```python
from build123d import *

# Parameters (mm, degrees)
SKETCH_W        = 10
SKETCH_H        = 6
PAD_DEPTH       = 3
SKETCH001_R     = 1.1
POCKET_DEPTH    = 6.001
SKETCH002_R     = 0.5
POCKET001_DEPTH = 1
CHAMFER_SIZE    = 1.2
SKETCH004_R     = 0.6
POCKET002_DEPTH = 6.001
FILLET_R        = 0.5
CHAMFER001_SIZE = 0.2


with BuildPart() as part:
    # Sketch → Pad (new body, symmetric)
    with BuildSketch(Plane.XY):
        with Locations((-5, 0)):
            Rectangle(SKETCH_W, SKETCH_H)
    extrude(amount=PAD_DEPTH, both=True)

    # Sketch001 (on Face6 of Pad) → Pocket (cut, through all)
    with BuildSketch(Plane.XY.offset(3)):
        with Locations((-5, 0)):
            Circle(SKETCH001_R)
    extrude(amount=-POCKET_DEPTH, mode=Mode.SUBTRACT)

    # Sketch002 (on Face1 of Pocket) → Pocket001 (cut)
    with BuildSketch(Plane.XZ.offset(3)):
        with Locations((-8.5, 0)):
            Circle(SKETCH002_R)
    extrude(amount=-POCKET001_DEPTH, mode=Mode.SUBTRACT)

    # Chamfer
    chamfer_edges = [part.edges().sort_by_distance(p)[0] for p in [
        (-6.1, 0, 3),
    ]]
    chamfer(chamfer_edges, length=CHAMFER_SIZE)

    # Sketch004 (on Face3 of Chamfer) → Pocket002 (cut, through all)
    with BuildSketch(Plane.XZ.offset(3)):
        with Locations((-8.5, 1.75)):
            Circle(SKETCH004_R)
        with Locations((-8.5, -1.75)):
            Circle(SKETCH004_R)
    extrude(amount=-POCKET002_DEPTH, mode=Mode.SUBTRACT)

    # Fillet
    fillet_edges = [part.edges().sort_by_distance(p)[0] for p in [
        (-10, 0, 3),
        (-10, 0, -3),
    ]]
    fillet(fillet_edges, radius=FILLET_R)

    # Mirrored: part across YZ


with BuildPart() as part_1:
    add(part.part)
    add(part.part.mirror(Plane.YZ))

    # Chamfer001
    chamfer001_edges = [part_1.edges().sort_by_distance(p)[0] for p in [
        (10, 3, 0),
        (0, -3, 3),
    ]]
    chamfer(chamfer001_edges, length=CHAMFER001_SIZE)


solid = part_1.part
```
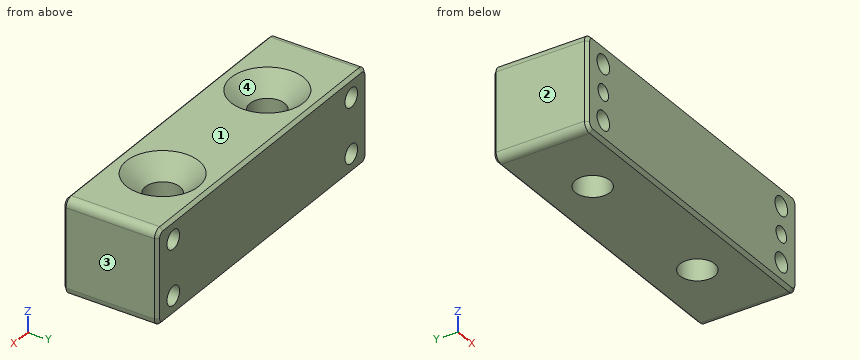
Input: part model. Units: mm. Frame: model coordinates. Face numbers are marked on the shaded views. Give positions to 0.01 mm unless a question says otherwise; leave off trailing zeros. Order: outer loops, then holes, each group sorted by start corner. A loop starts at its lowest first (then second) coordinate and runs counter-clockwise, first axis right, second up. Notation, with made-up numbers: M 76,-24 L 103,-24 A22 ccw 103,11 Z; hole C 40,1 d8. An arc over 180 degrees is marked long. One line per question, with ' | ' between items. Start each with the question number.
1. Section query C-C (y = 0). Return the cut outline in (x, z).
2. First-contact query: pin 1 Ø1.8 at (x, y) = (-5, 0) entering from -Z; pin 2 Ø3.5 at (x, y) = (5, 0) entering from +Z. Flat tips, straight axial feed; report the tip coordinate or a pass-through.
3. Section query A-A (z = -1.75). Return the cut outline in (x, y).
4. Section query D-D (x = -8.5). Return the cut outline in (y, z), and give its area (3 significant figures).
5. Pull-direction query (X, two-part tool) for the marked faces 1, 2, 3 and 4; classes: released by +X, released by -X, zero draft, split by the parting line, or undercut.
6. Section query B-B (x = 5). Return the cut outline in (y, z), and give its area (3 significant figures).
7. Material intervals for probe 1 along Z at (x, y) = (8.5, 0.45); probe 2 along X at (y, z) = (-0.25, -0.75); probe 3 along Y at (x, z) = (-8.5, -0.3), sorted ascending. Write a range as [from, to].
Here are the results:
1) outline: M -10,-2.5 A0.5 ccw -9.5,-3 L -6.1,-3 L -6.1,1.8 L -7.3,3 L -9.5,3 A0.5 ccw -10,2.5 Z; M -3.9,-3 L 3.9,-3 L 3.9,1.8 L 2.7,3 L -2.7,3 L -3.9,1.8 Z; M 6.1,-3 L 9.5,-3 A0.5 ccw 10,-2.5 L 10,2.5 A0.5 ccw 9.5,3 L 7.3,3 L 6.1,1.8 Z; hole C -8.5,-1.75 d1.2; hole C -8.5,1.75 d1.2; hole C 8.5,-1.75 d1.2; hole C 8.5,1.75 d1.2
2) pin 1: through | pin 2: z = 2.45
3) outline: M -10,-2.8 L -9.8,-3 L -9.1,-3 L -9.1,3 L -9.8,3 L -10,2.8 Z; M -7.9,-3 L 7.9,-3 L 7.9,3 L -7.9,3 Z; M 9.1,-3 L 9.8,-3 L 10,-2.8 L 10,2.8 L 9.8,3 L 9.1,3 Z; hole C -5,0 d2.2; hole C 5,0 d2.2
4) outline: M -3,-2.8 L -2.8,-3 L 2.8,-3 L 3,-2.8 L 3,-2.35 L -3,-2.35 Z; M -3,-1.15 L 3,-1.15 L 3,1.15 L -3,1.15 L -3,0.5 L -2,0.5 L -2,-0.5 L -3,-0.5 Z; M -3,2.35 L 3,2.35 L 3,2.8 L 2.8,3 L -2.8,3 L -3,2.8 Z | area: 20.5 mm²
5) face 1: zero draft | face 2: released by -X | face 3: released by +X | face 4: undercut
6) outline: M -3,-2.8 L -2.8,-3 L -1.1,-3 L -1.1,1.8 L -2.3,3 L -2.8,3 L -3,2.8 Z; M 1.1,-3 L 2.8,-3 L 3,-2.8 L 3,2.8 L 2.8,3 L 2.3,3 L 1.1,1.8 Z | area: 21.3 mm²
7) probe 1: [-3, -2.35], [-1.15, 1.15], [2.35, 3] | probe 2: [-10, -6.07], [-3.93, 3.93], [6.07, 10] | probe 3: [-2, 3]
